from build123d import *

# Parameters (mm, degrees)
F0_W     = 82.55
F0_H     = 44.45
F1_DEPTH = 19.05
F3_DEPTH = 41.402
F4_R     = 5.485136
F5_DEPTH = 6.35


with BuildPart() as f1:
    # F0 (on Top) → F1 (new body)
    with BuildSketch(Plane.XY):
        Rectangle(F0_W, F0_H)
    extrude(amount=F1_DEPTH)

    # F2 (on face) → F3 (cut)
    with BuildSketch(Plane(origin=(0, 22.225, 0), x_dir=(-1, 0, 0), z_dir=(0, 1, 0))):
        Polygon((36.041375, 14.287501), (-34.566533, 14.471854), (-34.566533, 3.963629), (36.041375, 3.963629), align=None)
    extrude(amount=-F3_DEPTH, mode=Mode.SUBTRACT)

    # F4 (on face) → F5 (cut)
    with BuildSketch(Plane.XY.offset(19.05)):
        with Locations((0, -13.734437)):
            Circle(F4_R)
    extrude(amount=-F5_DEPTH, mode=Mode.SUBTRACT)


solid = f1.part
Source: CAD feature listing. Evaluate the final solid. Frame: model axes, mm. A direction names the side the tool comes from. Coordinates: 2 decimals unless noted, no trailing zeros. Order: outer loops, then holes, each group sorted by start corner. A loop starts at its lowest first (then second) coordinate and runs counter-clockwise, first axis right, second up. Notation, with made-up numbers: M -29.75,70.5 L -20.75,70.5 A15 ccw -20.75,95.5 Z; hole C 56,79 d11. An arc over 180 degrees is marked long. Write each question's results on one line, items separated by ' | '. Start each with the question number.
1. Material intervals for L1, parallel to Z at x = 31, y = -18.5; L2, parallel to Z at x = -35, y = 13; L3, parallel to Y at x = 0, z = 15.75 (3 decimals), sorted ascending.
2. Pin query (flat end, axial travel): pin 1 (3 mm diameter, centred on x = -16, z = 7.5, fed in from +Y); pin 2 (6.5 mm diameter, centred on x = 0, y = -13.73, fed in from +Z). Return the tip coordinate at first contact, or that it passes through.
3. Draft query along X for faces 4 (the face through (-41.275, 0, 9)), 5 (the face through (41.275, 0, 9)), 6 (the face through (0, 2, 3.964)). Return one class per face: +X half, -X half, draft (parallel to the pull), parting line (faces both ways), or undercut.
4. Section C-C, the plane x = 26. Return the cut outline in (y, z) (3 decimals), then the cut area to 3 significant figures.
5. Reachability of faces 1 (the face through (-1, -22.225, 9)), 2 (the face through (-0.714, -8.296, 16.625)), 3 (the face through (34.567, 2, 9)) from +Z, -Z, +X, -X, +Y, -Y: full face, straight path, thin tool, end or side. Return the list, or none.
6. Section A-A, the plane x = 4.5. Return the cut outline in (y, z) (3 decimals).
7. Section D-D, the plane z = 16.5. Return the cut outline in (x, y) (3 decimals).
Solution:
1) L1: 0 to 3.96, 14.46 to 19.05 | L2: 0 to 3.96, 14.29 to 19.05 | L3: -22.225 to -19.22, -8.249 to 22.225
2) pin 1: y = -19.18 | pin 2: z = 3.96
3) face 4: -X half | face 5: +X half | face 6: undercut
4) outline: M -22.225,0 L 22.225,0 L 22.225,3.964 L -19.177,3.964 L -19.177,14.449 L 22.225,14.449 L 22.225,19.05 L -22.225,19.05 Z | area: 413 mm²
5) face 1: +Z, -Z, +X, -X, -Y | face 2: +Z | face 3: +Y
6) outline: M -22.225,0 L 22.225,0 L 22.225,3.964 L -19.177,3.964 L -19.177,14.393 L -16.871,14.393 L -16.871,19.05 L -22.225,19.05 Z; M -10.598,14.393 L 22.225,14.393 L 22.225,19.05 L -10.598,19.05 Z
7) outline: M -41.275,-22.225 L 41.275,-22.225 L 41.275,22.225 L -41.275,22.225 Z; hole C 0,-13.734 d10.97
